Source: CAD feature listing. Evaluate the final solid. Frame: model axes, mm. A direction names the side the tool comes from. Coordinates: 2 decimals unless noted, no trailing zeros. Order: outer loops, then holes, each group sorted by start corner. A loop starts at its lowest first (then second) coordinate and runs counter-clockwise, first axis right, second up. Notation, with made-up numbers: (8.5, 73) - (65.5, 73) arc R8 cw to (65.5, 87) - close; hole circle Ø5 at (5.5, -22). An arc over 180 degrees is marked (long way). One line per question, with ' | ' between items.
from build123d import *

# Parameters (mm, degrees)
SKETCH_1_R          = 14
EXTRUDE_1_DEPTH     = 4
SKETCH_2_R          = 6
CUT_EXTRUDE_1_DEPTH = 9
SKETCH_3_R          = 12.4
SKETCH_3_R_2        = 8.5
CUT_EXTRUDE_2_DEPTH = 0.5


with BuildPart() as part:
    # 草圖1 → 填料-伸長1 (new body, symmetric)
    with BuildSketch(Plane.XY):
        Circle(SKETCH_1_R)
    extrude(amount=EXTRUDE_1_DEPTH, both=True)

    # 草圖2 → 除料-伸長1 (cut, through all)
    with BuildSketch(Plane.XY.offset(4)):
        Circle(SKETCH_2_R)
    extrude(amount=-CUT_EXTRUDE_1_DEPTH, mode=Mode.SUBTRACT)

    # 草圖3 → 除料-伸長2 (cut)
    with BuildSketch(Plane.XY.offset(4)):
        Circle(SKETCH_3_R)
        Circle(SKETCH_3_R_2, mode=Mode.SUBTRACT)
    cut_extrude_2 = extrude(amount=-CUT_EXTRUDE_2_DEPTH, mode=Mode.SUBTRACT)

    # 鏡射1: 除料-伸長2 across plane
    add(cut_extrude_2.mirror(Plane.XY), mode=Mode.SUBTRACT)


solid = part.part
(1) Pull-direction query (X, two-part tool) for faces 4 (the flat face through (-2.1, -12.4, 4)), 5 (the flat face through (2.6, 8.4, 3.5)), 6 (the cylindrical face through (12.932, -5.362, 0.056)); classes: pulls with the +X half, pulls with the -X half, needs draft (parallel to the pull), parting line crosses it, or undercut.
Taken from the geometry:
face 4: needs draft | face 5: undercut | face 6: parting line crosses it
(2) Material intervals for L1, parallel to Y at x = 0, z = -3.85; L2, parallel to Z at x = 2.25, y = 9.75; L3, parallel to Y at x = 2.5, z = 0.75, sorted ascending. Write a range as from..to.
Taken from the geometry:
L1: y = -14..-12.4, -8.5..-6, 6..8.5, 12.4..14 | L2: z = -3.5..3.5 | L3: y = -13.77..-5.45, 5.45..13.77
(3) Set-up query: faces 1 (the cylindrical face through (4.57, 7.167, 3.754)), 2 (the cylindrical face through (5.72, -11, -3.75)), 3 (the cylindrical face through (-6, 0, 0)). Return all of +Z, -Z, +X, -X, +Y, -Y with unobstructed straight access to the full face (end or side cutting, diameter ignored); none if empty.
Taken from the geometry:
face 1: +Z | face 2: -Z | face 3: +Z, -Z
(4) Cut plane D-D (x = -7). Return the cut outline in (y, z), and give its area (3 significant figures).
Taken from the geometry:
outline: (-12.12, -4) - (-10.24, -4) - (-10.24, -3.5) - (-4.82, -3.5) - (-4.82, -4) - (4.82, -4) - (4.82, -3.5) - (10.24, -3.5) - (10.24, -4) - (12.12, -4) - (12.12, 4) - (10.24, 4) - (10.24, 3.5) - (4.82, 3.5) - (4.82, 4) - (-4.82, 4) - (-4.82, 3.5) - (-10.24, 3.5) - (-10.24, 4) - (-12.12, 4) - close | area: 183 mm²
(5) Pin query (flat end, axial travel): P1, Ø1.5, axis at x = -4.5, z = -2, coming from the -Y side. Return the tip coordinate at first contact, or that it passes through.
Taken from the geometry:
P1: stops at y = -13.49
(6) Cut plane A-A (x = 0). Return the cut outline in (y, z), and give its area (3 significant figures).
Taken from the geometry:
outline: (-14, -4) - (-12.4, -4) - (-12.4, -3.5) - (-8.5, -3.5) - (-8.5, -4) - (-6, -4) - (-6, 4) - (-8.5, 4) - (-8.5, 3.5) - (-12.4, 3.5) - (-12.4, 4) - (-14, 4) - close; (6, -4) - (8.5, -4) - (8.5, -3.5) - (12.4, -3.5) - (12.4, -4) - (14, -4) - (14, 4) - (12.4, 4) - (12.4, 3.5) - (8.5, 3.5) - (8.5, 4) - (6, 4) - close | area: 120 mm²
(7) Cut plane B-B (y = 1). Return the cut outline in (x, z), and give its area (3 significant figures).
Taken from the geometry:
outline: (-13.96, -4) - (-12.36, -4) - (-12.36, -3.5) - (-8.44, -3.5) - (-8.44, -4) - (-5.92, -4) - (-5.92, 4) - (-8.44, 4) - (-8.44, 3.5) - (-12.36, 3.5) - (-12.36, 4) - (-13.96, 4) - close; (5.92, -4) - (8.44, -4) - (8.44, -3.5) - (12.36, -3.5) - (12.36, -4) - (13.96, -4) - (13.96, 4) - (12.36, 4) - (12.36, 3.5) - (8.44, 3.5) - (8.44, 4) - (5.92, 4) - close | area: 121 mm²
(8) Cut plane C-C (z = 1.75). Return the cut outline in (x, y), and give its area (3 significant figures).
Taken from the geometry:
outline: circle Ø28 at (0, 0); hole circle Ø12 at (0, 0) | area: 503 mm²
